Here's the drawing with two shaded views (mm, measured from the low corner). I have some questions. A direction names the side the tool comes from. Round coordinates to 2 decimals unless told otherwise and drop trailing zeros. Order: outer loops, then holes, each group sorted by start corner. A loop starts at its lowest first (then second) coordinate and runs counter-clockwise, first axis right, second up. Notation, with made-up numbers: (-9, 3.25) -> (16, 3.25) arc R18 ccw to (16, 25.25) -> close; hole circle Ø1 at (-3.5, -30.5). An arc over 180 degrees is marked (long way). Put each result on its own line as item: value. Start each with the question number.
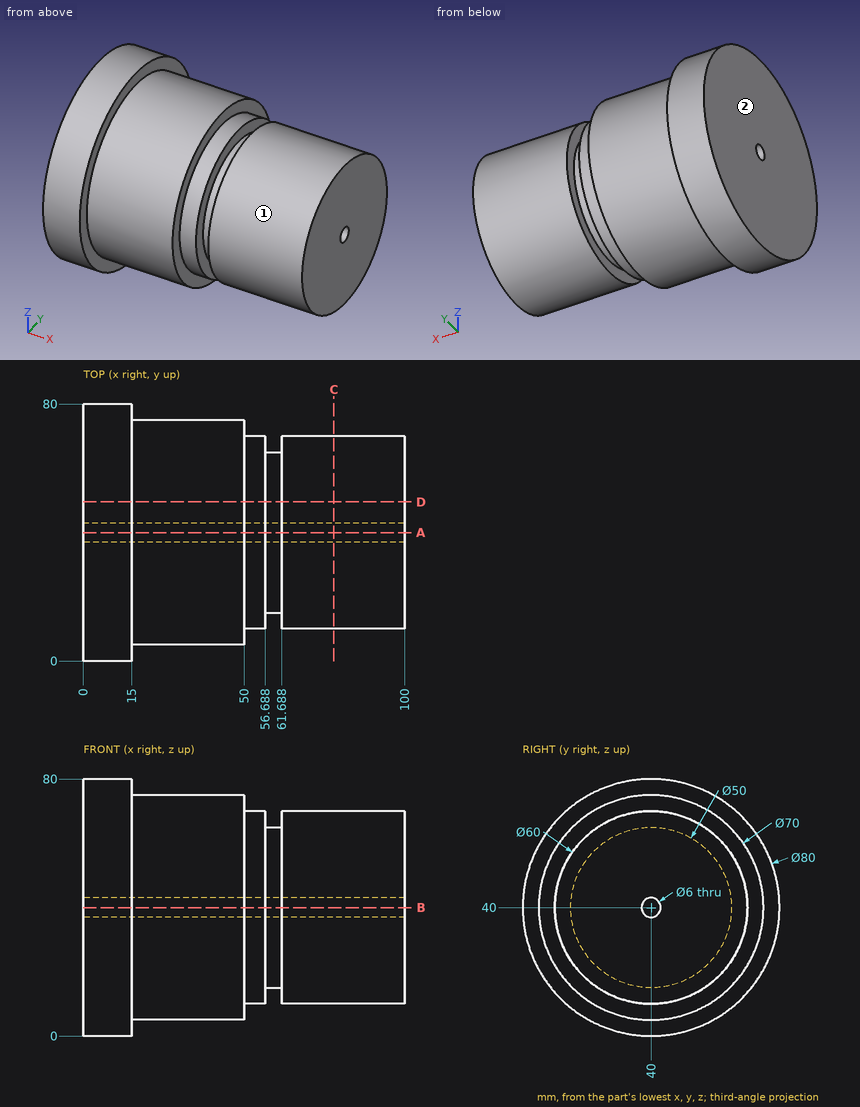
1. Which directions (+Z, -Z, +X, -X, +Y, -Y) give clear straight access to the entire face, cutting with the end or side of a thin tool? Please do the marked faces 1 and 2.
2. I need wall thicknesses on L1, parallel to Z at x = 15.5, y = 40; L2, parallel to Z at x = 51, y = 40; L3, parallel to X at y = 20, z = 62.5. Which ranges of each line are inside material? Lowest first, please.
3. If we section it at D-D, the plane y = 49.5: Please give me the cut outline in (x, z) (1 decimal), then the cut area to 3 significant figures.
4. For pin 1 Ø5 at (x, z) = (76, 26.5) entering from +Y; pin 2 Ø4 at (x, y) = (81.5, 32) entering from +Z; pin 3 Ø6 at (x, y) = (54, 19.5) entering from -Z, each with a flat end and sliding along its axis, tell me the tip position at first contact or that it passes through.
5. If we section it at A-A, the plane y = 40: Please give me the cut outline in (x, z).
6. If we section it at C-C, the plane x = 78: Please give me the cut outline in (y, z).
Results below:
1. face 1: +X
1. face 2: +Z, -Z, -X, +Y, -Y
2. L1: 5 to 37, 43 to 75
2. L2: 10 to 37, 43 to 70
2. L3: 0 to 50
3. outline: (0, 1.1) -> (15, 1.1) -> (15, 6.3) -> (50, 6.3) -> (50, 11.5) -> (56.7, 11.5) -> (56.7, 16.9) -> (61.7, 16.9) -> (61.7, 11.5) -> (100, 11.5) -> (100, 68.5) -> (61.7, 68.5) -> (61.7, 63.1) -> (56.7, 63.1) -> (56.7, 68.5) -> (50, 68.5) -> (50, 73.7) -> (15, 73.7) -> (15, 78.9) -> (0, 78.9) -> close
3. area: 6,320 mm2
4. pin 1: y = 67.91
4. pin 2: z = 69.39
4. pin 3: z = 15.63
5. outline: (0, 0) -> (15, 0) -> (15, 5) -> (50, 5) -> (50, 10) -> (56.69, 10) -> (56.69, 15) -> (61.69, 15) -> (61.69, 10) -> (100, 10) -> (100, 37) -> (0, 37) -> close; (0, 43) -> (100, 43) -> (100, 70) -> (61.69, 70) -> (61.69, 65) -> (56.69, 65) -> (56.69, 70) -> (50, 70) -> (50, 75) -> (15, 75) -> (15, 80) -> (0, 80) -> close
6. outline: circle Ø60 at (40, 40); hole circle Ø6 at (40, 40)
